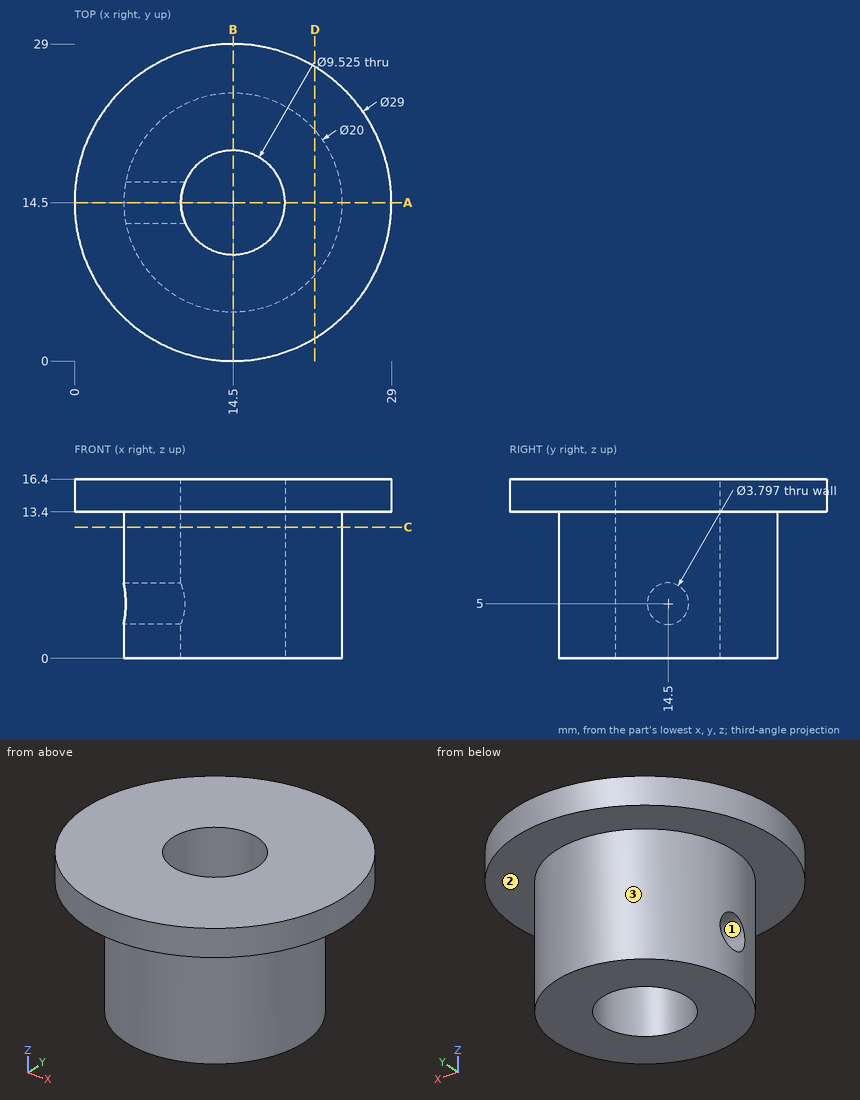
Answer from the drawing. Dimensions are ordinates in mm from the lowest x, y and z of the part. Give positions to 0.01 mm unless a question says otherwise; leave off trailing zeros. Order: outer loops, then holes, each group sorted by start corner. A loop starts at its lowest first (then second) coordinate and runs counter-clockwise, first axis right, second up. Notation, with made-up numbers: (1.25, -38.5) -> (29.25, -38.5) arc R24 cw to (29.25, -9.5) -> close; hole circle Ø5 at (45, 75.5). An arc over 180 degrees is marked (long way). One line per item, written item: value. Start each with the question number.
(1) The part is cut by section B-B (x = 14.5). Determine the outline of the cut face in (y, z).
(2) The part is cut by section D-D (x = 22). Determine the outline of the cut face in (y, z).
(3) Straight lines are drawn through the part: L1, parallel to X at y = 14.5, z = 8.25; L2, parallel to Z at x = 13.5, y = 26.25. For each, find the intervals that lie inside material, in ascending order.
(4) Flat-ended cylindrical pins translate along their axes: P1, Ø4, axis at x = 10, z = 3, coming from the +Y side; P2, Ø2.5, axis at y = 14.5, z = 5, coming from the +X side; P3, Ø2, axis at y = 8.5, z = 12.5, coming from the -X side. Find the tip coordinate at first contact, or state that the pin passes through.
(5) For a pull along Y with two mould halves and no side action, classify the marked faces 1, 2 and 3 as released by +Y, released by -Y, zero draft, split by the parting line, or undercut.
(6) The part is cut by section C-C (z = 12). Determine the outline of the cut face in (x, y) (1 decimal).
(7) The part is cut by section A-A (y = 14.5). Determine the outline of the cut face in (x, z), and give its area (3 significant figures).
Taken from the geometry:
1. outline: (0, 13.4) -> (4.5, 13.4) -> (4.5, 0) -> (9.74, 0) -> (9.74, 16.4) -> (0, 16.4) -> close; (19.26, 0) -> (24.5, 0) -> (24.5, 13.4) -> (29, 13.4) -> (29, 16.4) -> (19.26, 16.4) -> close
2. outline: (2.09, 13.4) -> (7.89, 13.4) -> (7.89, 0) -> (21.11, 0) -> (21.11, 13.4) -> (26.91, 13.4) -> (26.91, 16.4) -> (2.09, 16.4) -> close
3. L1: 4.5 to 9.74, 19.26 to 24.5
3. L2: 13.4 to 16.4
4. P1: y = 24.18
4. P2: x = 24.5
4. P3: x = 1.11
5. face 1: undercut
5. face 2: zero draft
5. face 3: split by the parting line
6. outline: circle Ø20 at (14.5, 14.5); hole circle Ø9.5 at (14.5, 14.5)
7. outline: (0, 13.4) -> (4.5, 13.4) -> (4.5, 6.9) -> (9.74, 6.9) -> (9.74, 16.4) -> (0, 16.4) -> close; (4.5, 0) -> (9.74, 0) -> (9.74, 3.1) -> (4.5, 3.1) -> close; (19.26, 0) -> (24.5, 0) -> (24.5, 13.4) -> (29, 13.4) -> (29, 16.4) -> (19.26, 16.4) -> close
7. area: 179 mm^2
